```python
from build123d import *

# Parameters (mm, degrees)
BOSS_EXTRUDE1_DEPTH = 18.575
SKETCH3_R           = 2.5
CUT_EXTRUDE1_DEPTH  = 39.395420734


with BuildPart() as part:
    # Sketch2 → Boss-Extrude1 (new, symmetric)
    with BuildSketch(Plane(origin=(0, 0, 0), x_dir=(0, 0, -1), z_dir=(1, 0, 0))):
        Polygon((7.332348419, 0), (3.666174209, 6.35), (-3.666174209, 6.35), (-7.332348419, 0), (-3.666174209, -6.35), (3.666174209, -6.35), align=None)
    extrude(amount=BOSS_EXTRUDE1_DEPTH, both=True)

    # Sketch3 → Cut-Extrude1 (cut, through all)
    with BuildSketch(Plane.ZY.offset(18.575)):
        Circle(SKETCH3_R)
    extrude(amount=-CUT_EXTRUDE1_DEPTH, mode=Mode.SUBTRACT)


solid = part.part
```
Geometry: final body of the model. Coordinates: model frame, mm. Round coordinates to 2 decimals unless told otherwise and drop trailing zeros. Order: outer loops, then holes, each group sorted by start corner. A loop starts at its lowest first (then second) coordinate and runs counter-clockwise, first axis right, second up. Notation, with made-up numbers: (33, 29) - (37, 29) arc R25 cw to (37, 49) - close; hole circle Ø6 at (57, 87.5). An arc over 180 degrees is marked (long way). Write item = value, one per line. Start each with the question number.
Q1. Cut plane A-A on z = 0. Return the cut outline in (x, y) (3 decimals).
Q2. Cut plane B-B on y = 1.25. Return the cut outline in (x, z) (3 decimals).
Q3. Ray query, line 1 (Y direction, x = -3.5, z = 0); line 2 (Z direction, x = 6, y = 2); line 3 (Y direction, x = -5.5, z = 1). Return the intervals inside material, ascending. Write a range as from..to.
Q4. Pull-direction query (Y, two-part tool) for faces 1 (the flat face through (0.26, -3.131, 5.525)), 2 (the flat face through (0.26, 3.219, 5.474)), 3 (the flat face through (18.575, 0, -3)), 4 (the cylindrical face through (-0.26, -2.44, -0.54)); classes: +Y half, -Y half, draft (parallel to the pull), parting line (faces both ways), or undercut.
Q5. Cut plane D-D on z = -5.25. Return the cut outline in (x, y) (3 decimals).
Q6. Pin query (flat end, axial travel): pin 1 (6 mm diameter, centred on x = 12, z = -5, fed in from -Y); pin 2 (3 mm diameter, centred on x = 13, z = -5.5, fed in from +Y); pin 3 (3 mm diameter, centred on y = 0, z = 0, fed in from +X). Return the tip coordinate at first contact, or that it passes through.
Q7. Cut plane C-C on x = 8. Return the cut outline in (y, z).
Outcome:
q1.outline = (-18.575, -6.35) - (18.575, -6.35) - (18.575, -2.5) - (-18.575, -2.5) - close; (-18.575, 2.5) - (18.575, 2.5) - (18.575, 6.35) - (-18.575, 6.35) - close
q2.outline = (-18.575, -6.611) - (18.575, -6.611) - (18.575, -2.165) - (-18.575, -2.165) - close; (-18.575, 2.165) - (18.575, 2.165) - (18.575, 6.611) - (-18.575, 6.611) - close
q3.line_1 = -6.35..-2.5, 2.5..6.35
q3.line_2 = -6.18..-1.5, 1.5..6.18
q3.line_3 = -6.35..-2.29, 2.29..6.35
q4.face_1 = -Y half
q4.face_2 = +Y half
q4.face_3 = draft
q4.face_4 = undercut
q5.outline = (-18.575, -3.607) - (18.575, -3.607) - (18.575, 3.607) - (-18.575, 3.607) - close
q6.pin_1 = -6.35
q6.pin_2 = 5.77
q6.pin_3 = through
q7.outline = (-6.35, -3.67) - (0, -7.33) - (6.35, -3.67) - (6.35, 3.67) - (0, 7.33) - (-6.35, 3.67) - close; hole circle Ø5 at (0, 0)
